```python
from build123d import *

# Parameters (mm, degrees)
BOSS_EXTRUDE2_DEPTH = 50
BOSS_EXTRUDE3_DEPTH = 15


with BuildPart() as part:
    # Sketch1 → Boss-Extrude2 (new body)
    with BuildSketch(Plane(origin=(0, 0, 0), x_dir=(1, 0, 0), z_dir=(0, 1, 0))):
        Polygon((13.5, -22.5), (-13.5, -22.5), (-13.5, 22.5), (-15.1, 22.5), (-15.1, -24.1), (15.1, -24.1), (15.1, 34.1), (-15.1, 34.1), (-15.1, 32.5), (13.5, 32.5), align=None)
    extrude(amount=BOSS_EXTRUDE2_DEPTH)

    # Sketch1<4> → Boss-Extrude3 (add)
    with BuildSketch(Plane(origin=(0, 0, 0), x_dir=(1, 0, 0), z_dir=(0, 1, 0))):
        Polygon((13.5, 32.5), (13.5, -22.5), (-13.5, -22.5), (-13.5, 22.5), (-15.1, 22.5), (-15.1, -24.1), (15.1, -24.1), (15.1, 34.1), (-15.1, 34.1), (-15.1, 32.5), align=None)
        Polygon((-13.5, -22.5), (13.5, -22.5), (13.5, 32.5), (-15.1, 32.5), (-15.1, 22.5), (-13.5, 22.5), align=None)
    extrude(amount=BOSS_EXTRUDE3_DEPTH)


solid = part.part
```
Can you work these out from the model? Positions are in its coordinate system, mm. A direction names the side the tool comes from. Round coordinates to 2 decimals unless told otherwise and drop trailing zeros. Loops run counter-clockwise (first coordinate to the right, second up) from the corner with the lowest first, then second, coordinate; pieces in that order, holes last.
Item 1: Suppose I cut it at D-D, the plane z = -30. Write out the boundary of the cut face in (x, y), then the cut area to 3 significant figures.
Item 2: Will this pin go through, and if not, where does the flat tip stop? pin 1 Ø2 at (x, z) = (-5.5, -12.5) entering from +Y.
Item 3: Which directions (+Z, -Z, +X, -X, +Y, -Y) give clear straight access to the entire face, cutting with the end or side of a thin tool? Please do faces 4 (the flat face through (-1, 32, -32.5)), 5 (the flat face through (-13.5, 32, 0)), 6 (the flat face through (14, 50, -5)).
Item 4: Suppose I cut it at B-B, the plane y = 29.5. Write out the boundary of the cut face in (x, z).
Item 5: If we mould it in two halves opening along Z, with no side actions, what happens to faces 1 (the flat face through (-14, 32, -22.5)), 2 (the flat face through (0, 0, -5)), 3 (the flat face through (0, 25, -34.1))? For each: +Z half, -Z half, draft (parallel to the pull), parting line (faces both ways), or undercut.
Item 6: Suppose I cut it at C-C, the plane x = 3.5. Write out the boundary of the cut face in (y, z), then the cut area to 3 significant figures.
Item 7: Suppose I cut it at A-A, the plane z = 15. Write out the boundary of the cut face in (x, y).
Item 8: Please list where these lines run through material, in increasing order: L1, parallel to Z at x = -6, y = 16; L2, parallel to X at y = 47, z = 14.5; L3, parallel to Y at x = -8, z = 1.5.
Reported:
1. outline: (-15.1, 0) - (15.1, 0) - (15.1, 50) - (13.5, 50) - (13.5, 15) - (-15.1, 15) - close
1. area: 509 mm2
2. pin 1: stops at y = 15
3. face 4: -X, +Y
3. face 5: +Y
3. face 6: +Z, -Z, +X, -X, +Y
4. outline: (-15.1, -34.1) - (15.1, -34.1) - (15.1, 24.1) - (-15.1, 24.1) - (-15.1, -22.5) - (-13.5, -22.5) - (-13.5, 22.5) - (13.5, 22.5) - (13.5, -32.5) - (-15.1, -32.5) - close
5. face 1: undercut
5. face 2: draft
5. face 3: -Z half
6. outline: (0, -34.1) - (50, -34.1) - (50, -32.5) - (15, -32.5) - (15, 22.5) - (50, 22.5) - (50, 24.1) - (0, 24.1) - close
6. area: 985 mm2
7. outline: (-15.1, 0) - (15.1, 0) - (15.1, 50) - (13.5, 50) - (13.5, 15) - (-13.5, 15) - (-13.5, 50) - (-15.1, 50) - close
8. L1: z = -34.1 to -32.5, 22.5 to 24.1
8. L2: x = -15.1 to -13.5, 13.5 to 15.1
8. L3: y = 0 to 15
